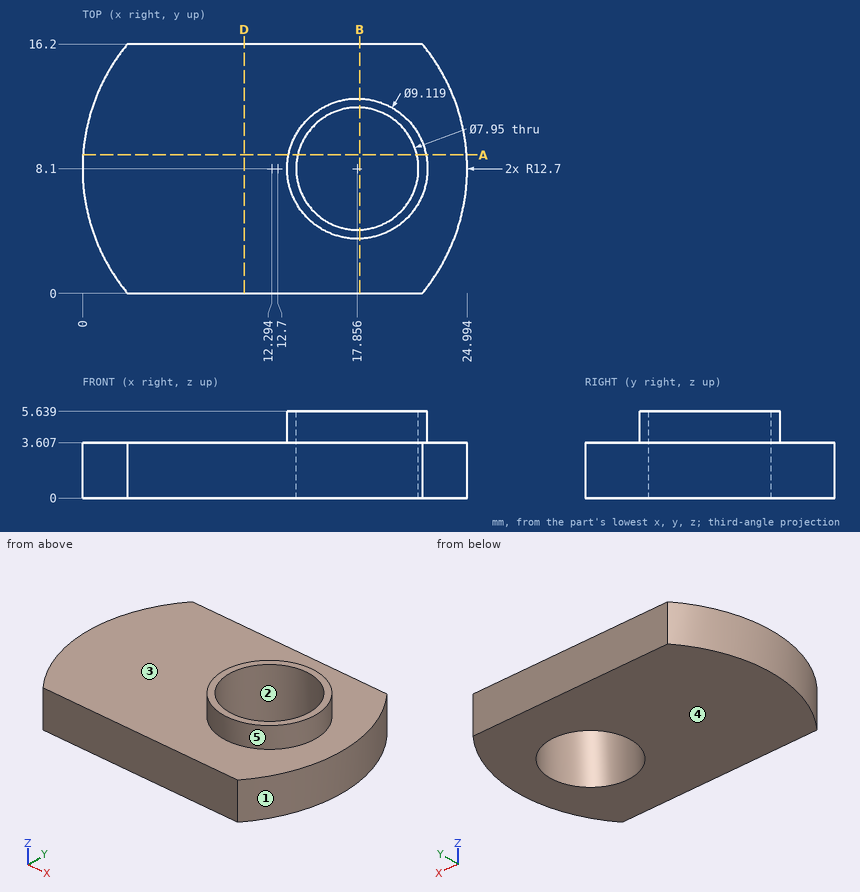
Design review of the part shown in the three views and the two pictorial views. Dimensions are in mm from the part's minimum x, y and z. A direction names the side the tool comes from. Round coordinates to 2 decimals unless told otherwise and drop trailing zeros. Loops run counter-clockwise (first coordinate to the right, second up) from the corner with the lowest first, then second, coordinate; pieces in that order, holes last. Notation, with made-up numbers: (77.5, 80) - (123.5, 80) arc R18 ccw to (123.5, 105) - close; hole circle Ø5 at (-20, 70). An arc over 180 degrees is marked (long way). Use CSV: the item, a comma, the result in double quotes.
(1) Take a section at D-D, the plane x = 10.5. Give the boundary of the cut face in (y, z).
Working result:
outline,"(0, 0) - (16.2, 0) - (16.2, 3.61) - (0, 3.61) - close"
(2) Clearance check with a flat-ended pin moving along its axis: P1, Ø2, axis at y = 11, z = 4, coming from the +X side. State where the tip first meets the part, or that it passes through.
Working result:
P1,"stops at x = 24.84"
(3) Take a section at A-A, the plane y = 9. Give the boundary of the cut face in (x, z) (1 decimal).
Working result:
outline,"(0, 0) - (14, 0) - (14, 5.6) - (13.4, 5.6) - (13.4, 3.6) - (0, 3.6) - close; (21.7, 0) - (25, 0) - (25, 3.6) - (22.3, 3.6) - (22.3, 5.6) - (21.7, 5.6) - close"
(4) Machinability: for the marked faces 4 and 5, which of the approach directions +Z, -Z, +X, -X, +Y, -Y give a long, thin tool a straight path to every point of the face, cutting with its end or side? Answer none if there is none.
Working result:
face 4,"-Z, +X, -X, +Y, -Y"
face 5,"+Z"
(5) The part is to be moulded in two halves that separate along Y. For the marked faces 1, 2 and 3, say which applies: pulls with the +Y half, pulls with the -Y half, needs draft (parallel to the pull), parting line crosses it, or undercut.
Working result:
face 1,"parting line crosses it"
face 2,"undercut"
face 3,"needs draft"
(6) Take a section at B-B, the plane x = 18. Give the boundary of the cut face in (y, z).
Working result:
outline,"(0, 0) - (4.13, 0) - (4.13, 5.64) - (3.54, 5.64) - (3.54, 3.61) - (0, 3.61) - close; (12.07, 0) - (16.2, 0) - (16.2, 3.61) - (12.66, 3.61) - (12.66, 5.64) - (12.07, 5.64) - close"
(7) For line 1 (X direction, y = 11, z = 5.3) (1 decimal); line 2 (Z direction, x = 11.5, y = 5); line 3 (X direction, y = 8.75, z = 0.95) (1 decimal), list the stretches that pass through material, from the lowest coordinate up.
Working result:
line 1,"x = 14.3 to 15.1, 20.6 to 21.4"
line 2,"z = 0 to 3.61"
line 3,"x = 0 to 13.9, 21.8 to 25"
